The drawing under review shows one solid part. Ordinate dimensions are in mm from its lowest x, y, z. Round coordinates to 2 decimals unless told otherwise and drop trailing zeros. Write each loop counter-clockwise with the first axis right and the second up, starting at its lowest first coordinate (ties: lowest second). Pieces come first, ordered by that corner, then holes.
Item 1: Clearance check with flat-ended pins moving along their axes: pin 1 Ø3 at (y, z) = (8.5, 14) entering from +X; pin 2 Ø5 at (x, y) = (5, 1.5) entering from -Z; pin 3 Ø12 at (x, z) = (20.5, 3.5) entering from +Y; pin 4 Ø3 at (x, y) = (8, 1) entering from +Z. State where each tip first meets the part, or that it passes through.
Item 2: Add section D-D (y = 7). Give the boundary of the cut face in (x, z), plus the area to 3 significant figures.
Item 3: Add section C-C (y = 1.5). Give the boundary of the cut face in (x, z).
Item 4: To check wall thickness, follow L1, parallel to X at y = 7.9, z = 12; L2, parallel to Z at x = 16, y = 5.5. State the ranges of each line that lie inside material, in increasing order.
Item 5: Add section A-A (z = 12). Give the boundary of the cut face in (x, y), plus the area to 3 significant figures.
Item 6: Add section B-B (x = 12). Give the boundary of the cut face in (y, z), plus the area to 3 significant figures.
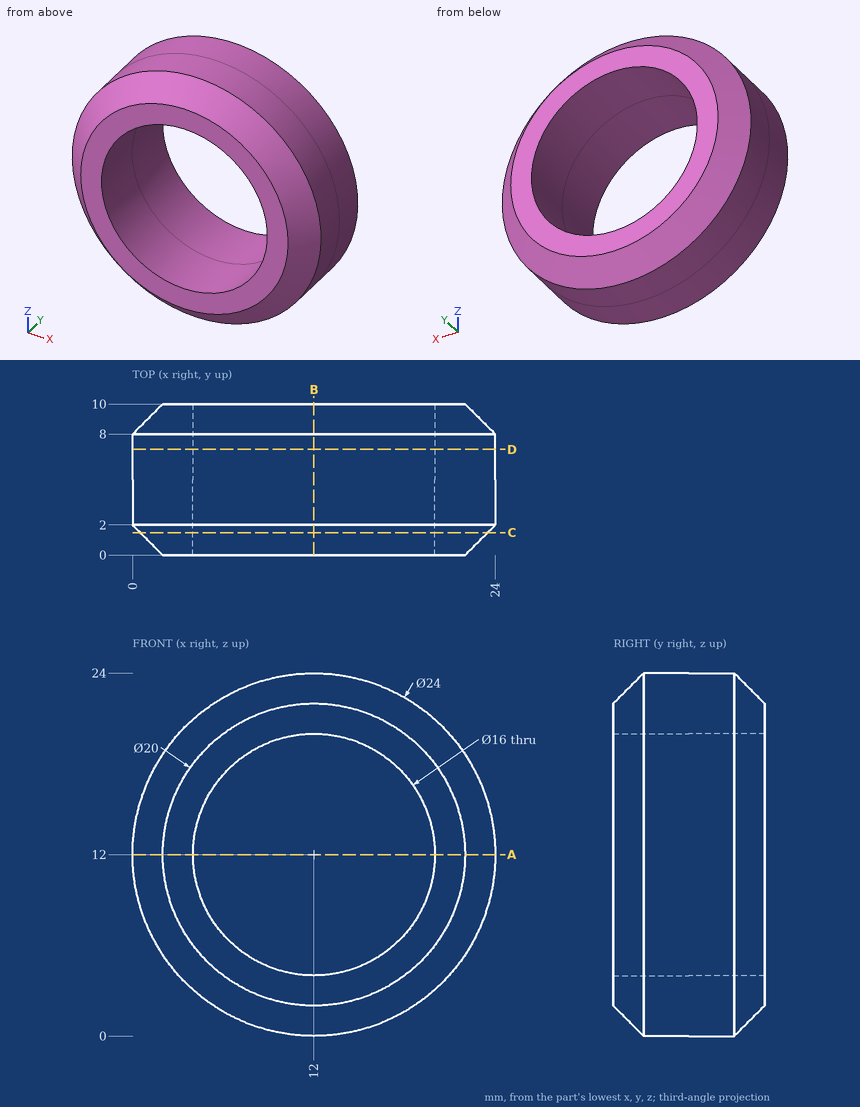
Numbers:
1. pin 1: stops at x = 23.99
1. pin 2: stops at z = 0.9
1. pin 3: stops at y = 10
1. pin 4: stops at z = 23.65
2. outline: circle Ø24 at (12, 12); hole circle Ø16 at (12, 12)
2. area: 251 mm2
3. outline: circle Ø23 at (12, 12); hole circle Ø16 at (12, 12)
4. L1: x = 0 to 4, 20 to 24
4. L2: z = 0.69 to 5.07, 18.93 to 23.31
5. outline: (0, 2) - (2, 0) - (4, 0) - (4, 10) - (2, 10) - (0, 8) - close; (20, 0) - (22, 0) - (24, 2) - (24, 8) - (22, 10) - (20, 10) - close
5. area: 72.0 mm2
6. outline: (0, 2) - (2, 0) - (8, 0) - (10, 2) - (10, 4) - (0, 4) - close; (0, 20) - (10, 20) - (10, 22) - (8, 24) - (2, 24) - (0, 22) - close
6. area: 72.0 mm2
